For this review, take the finished solid that the model builds, in its own axes (mm). A direction names the side the tool comes from. Give positions to 0.01 mm unless a question says otherwise; leave off trailing zeros. Write each loop counter-clockwise with the first axis right and the second up, starting at its lowest first coordinate (ties: lowest second). Pieces come first, ordered by that corner, then holes.
Q1. We need section A-A (z = 1.6). Write out the cut boundary in (x, y).
Q2. We need section B-B (x = -5). Write out the cut boundary in (y, z), then the cut area to 3 significant figures.
Q3. We need section C-C (z = -0.9). Write out the cut boundary in (x, y), then the cut area to 3 significant figures.
Q4. We need section D-D (x = -6.5). Write out the cut boundary in (y, z).
Q5. Machinability: for faces 5 (the flat face through (-6, 1.25, 1)), 6 (the cylindrical face through (-1.825, -1.4, -3.014)), 7 (the cylindrical face through (-2.56, 2.08, -2.03)), 8 (the cylindrical face through (-1.825, -1.4, 1.493)), which of the approach directions +Z, -Z, +X, -X, +Y, -Y give a long, thin tool a straight path to every point of the face, cutting with its end or side? Answer none if there is none.
Q6. Insertion check: P1, Ø3.5, axis at x = 0, y = 0, coming from the +Z side; P2, Ø1.2, axis at x = 0, y = 0, coming from the -Z side; P3, Ø3, axis at x = 0, y = 0, coming from the -Z side; P4, Ø3, axis at x = -5, y = 0.5, coming from the -Z side. Each pin has a flat end and moves straight along its axis. Give the tip position at first contact, or say it passes through.
Q7. Mouldability with a two-part tool opening along Y and no side actions: class faces 1 (the flat face through (-1, -1, -2)), 2 (the flat face through (2, 2, -4)), 3 (the cylindrical face through (-8.75, 0.04, 0.99)), 4 (the cylindrical face through (-2.587, -2.049, -2.028)) as released by +Y, released by -Y, zero draft, split by the parting line, or undercut.
Q8. For line 1 (Z direction, x = -4, y = 2); line 2 (Y direction, x = 1, z = -2.65); line 3 (Y direction, x = -1.5, z = -3.1), list the stretches that pass through material, from the lowest coordinate up.
```python
from build123d import *

# Parameters (mm, degrees)
SKIZZE1_R                       = 2.3
AUFSATZ_LINEAR_AUSTRAGEN1_DEPTH = 2
AUFSATZ_LINEAR_START            = -4
SKIZZE1_11_R                    = 2.3
AUFSATZ_LINEAR_AUSTRAGEN2_DEPTH = 4
AUFSATZ_LINEAR_START_2          = -2
SKIZZE1_13_R                    = 2.3
SKIZZE1_13_R_2                  = 1
AUFSATZ_LINEAR_AUSTRAGEN3_DEPTH = 2
VERRUNDUNG1_R                   = 1


with BuildPart() as part:
    # Skizze1 → Aufsatz-Linear austragen1 (new body)
    with BuildSketch(Plane.XY):
        with BuildLine():
            ThreePointArc((-7, 1.75), (-8.75, 0), (-7, -1.75))
            Line((-7, -1.75), (0, -3.3))
            ThreePointArc((0, -3.3), (3.3, 0), (0, 3.3))
            Line((0, 3.3), (-7, 1.75))
        make_face()
        with BuildLine():
            ThreePointArc((-4.25, 1.25), (-3, 0), (-4.25, -1.25))
            Line((-4.25, -1.25), (-7, -1.25))
            ThreePointArc((-7, -1.25), (-8.25, 0), (-7, 1.25))
            Line((-7, 1.25), (-4.25, 1.25))
        make_face(mode=Mode.SUBTRACT)
        Circle(SKIZZE1_R, mode=Mode.SUBTRACT)
    extrude(amount=AUFSATZ_LINEAR_AUSTRAGEN1_DEPTH)

    # Skizze1<11> → Aufsatz-Linear austragen2 (add)
    with BuildSketch(Plane.XY.offset(AUFSATZ_LINEAR_START)):
        with BuildLine():
            Line((0, 3.3), (-1.393122903, 2.991522786))
            ThreePointArc((-1.393122903, 2.991522786), (-2.57392942, 2.065160367), (-3.222352941, 0.711647049))
            ThreePointArc((-3.222352941, 0.711647049), (-3, 0), (-3.222352941, -0.711647049))
            ThreePointArc((-3.222352941, -0.711647049), (-2.57392942, -2.065160367), (-1.393122903, -2.991522786))
            Line((-1.393122903, -2.991522786), (0, -3.3))
            ThreePointArc((0, -3.3), (2.333452378, -2.333452378), (3.3, 0))
            ThreePointArc((3.3, 0), (2.333452378, 2.333452378), (0, 3.3))
        make_face()
        Circle(SKIZZE1_11_R, mode=Mode.SUBTRACT)
    extrude(amount=AUFSATZ_LINEAR_AUSTRAGEN2_DEPTH)

    # Skizze1<13> → Aufsatz-Linear austragen3 (add)
    with BuildSketch(Plane.XY.offset(AUFSATZ_LINEAR_START_2)):
        Circle(SKIZZE1_13_R)
        Circle(SKIZZE1_13_R_2, mode=Mode.SUBTRACT)
    extrude(amount=AUFSATZ_LINEAR_AUSTRAGEN3_DEPTH)

    # Verrundung1
    verrundung1_edges = [part.edges().sort_by_distance(p)[0] for p in [
        (-2.3, 0, 0),
    ]]
    fillet(verrundung1_edges, radius=VERRUNDUNG1_R)


solid = part.part
```
Computed:
1. outline: (-7, -1.75) - (0, -3.3) arc R3.3 ccw to (0, 3.3) - (-7, 1.75) arc R1.75 ccw to start; hole (-7, -1.25) - (-4.25, -1.25) arc R1.25 ccw to (-4.25, 1.25) - (-7, 1.25) arc R1.25 ccw to start; hole circle Ø4.6 at (0, 0)
2. outline: (-2.19, 0) - (-1.25, 0) - (-1.25, 2) - (-2.19, 2) - close; (1.25, 0) - (2.19, 0) - (2.19, 2) - (1.25, 2) - close
2. area: 3.77 mm2
3. outline: (-3.22, -0.71) arc R3.3 ccw to (-1.39, -2.99) - (0, -3.3) arc R3.3 ccw to (0, 3.3) - (-1.39, 2.99) arc R3.3 ccw to (-3.22, 0.71) arc R1.25 cw to start; hole circle Ø2 at (0, 0)
3. area: 30.6 mm2
4. outline: (-1.86, 0) - (-1.25, 0) - (-1.25, 2) - (-1.86, 2) - close; (1.25, 0) - (1.86, 0) - (1.86, 2) - (1.25, 2) - close
5. face 5: +Z, -Z
5. face 6: -Z
5. face 7: -Z, -X, +Y
5. face 8: +Z
6. P1: stops at z = 0.11
6. P2: passes through
6. P3: stops at z = -2
6. P4: stops at z = 0
7. face 1: undercut
7. face 2: zero draft
7. face 3: split by the parting line
7. face 4: released by -Y
8. line 1: z = 0 to 2
8. line 2: y = -3.14 to -2.07, 2.07 to 3.14
8. line 3: y = -2.94 to -1.74, 1.74 to 2.94
